Verification items for the finished model (mm, model axes). Coordinates: 2 decimals unless noted, no trailing zeros. Write each loop counter-clockwise with the first axis right and the second up, starting at its lowest first coordinate (ties: lowest second). Pieces come first, ordered by that corner, then holes. Notation, with made-up numbers: (-0.75, 52) -> (32.25, 52) arc R7 cw to (32.25, 61) -> close; hole circle Ø6 at (38, -9). An arc over 180 degrees is marked (long way). Write item = value, one per line. Start each with the question number.
(1) Gauge pin test, flat ends, axial feed: pin 1 Ø1.5 at (x, y) = (46.5, 2) entering from +Z; pin 2 Ø10 at (x, z) = (-20.5, 9) entering from -Y; pin 3 Ø0.8 at (x, y) = (93.5, 3) entering from +Z; pin 4 Ø2 at (x, y) = (74.5, 4) entering from -Z. Record the tip position at first contact, or that the pin passes through.
(2) Section check B-B (y = 6.5). State how many separate pieces and enclosed holes the cut face has, plus the area to 3 significant figures.
(3) Section check A-A (x = 58.5). Record the cut outline in (y, z), plus the area to 3 significant figures.
(4) Material ranges on probe 1 along X at (y, z) = (7.3, 0); probe 2 along X at (y, z) = (8, -33.5); probe 3 along Z at (x, y) = (-19, 4.5), recorded low to high. Write a range as [from, to].
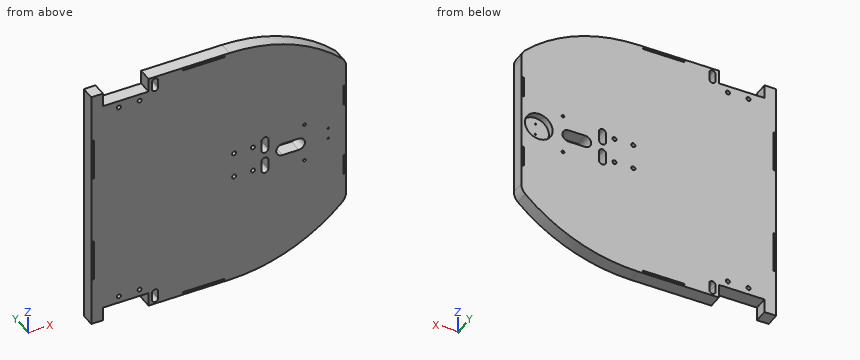
```python
from build123d import *

# Parameters (mm, degrees)
BOSS_EXTRUDE1_DEPTH = 10
SKETCH2_R           = 1
SKETCH2_R_2         = 1.5
SKETCH2_W           = 33
SKETCH2_H           = 10
CUT_EXTRUDE2_DEPTH  = 15
SKETCH3_R           = 10
CUT_EXTRUDE3_DEPTH  = 5
CUT_EXTRUDE4_DEPTH  = 15
SKETCH5_W           = 30
SKETCH5_H           = 1
SKETCH5_W_2         = 1
SKETCH5_H_2         = 30
SKETCH5_H_3         = 15
CUT_EXTRUDE6_DEPTH  = 15
SKETCH6_R           = 0.5
CUT_EXTRUDE7_DEPTH  = 15
SKETCH7_R           = 1.5
CUT_EXTRUDE8_DEPTH  = 132.376296717


with BuildPart() as part:
    # Sketch1 → Boss-Extrude1 (new body)
    with BuildSketch(Plane(origin=(0, 0, 0), x_dir=(1, 0, 0), z_dir=(0, 1, 0))):
        with BuildLine():
            Line((-89.389143795, -90), (-89.389143795, 90))
            Line((-89.389143795, 90), (10.610856205, 90))
            ThreePointArc((10.610856205, 90), (54.533138364, 81.496268076), (92.107774725, 57.214031174))
            ThreePointArc((92.107774725, 57.214031174), (94.381847518, 53.920998768), (95.182620993, 50))
            Line((95.182620993, 50), (95.182620993, -50))
            ThreePointArc((95.182620993, -50), (94.381847518, -53.920998768), (92.107774725, -57.214031174))
            ThreePointArc((92.107774725, -57.214031174), (54.533138364, -81.496268076), (10.610856205, -90))
            Line((10.610856205, -90), (-89.389143795, -90))
        make_face()
    extrude(amount=BOSS_EXTRUDE1_DEPTH)

    # Sketch2 → Cut-Extrude2 (cut, symmetric)
    with BuildSketch(Plane(origin=(0, 10, 0), x_dir=(1, 0, 0), z_dir=(0, 1, 0))):
        with Locations(Location((65, 14.131573434, 0), (0, 0, 90))):
            Circle(SKETCH2_R)
        with Locations(Location((27.688972694, 9.173126615, 0), (0, 0, 90))):
            Circle(SKETCH2_R_2)
        with Locations(Location((14.053243942, 9.173126615, 0), (0, 0, 90))):
            Circle(SKETCH2_R_2)
        with Locations(Location((14.053243942, -9.173126615, 0), (0, 0, 90))):
            Circle(SKETCH2_R_2)
        with Locations(Location((27.688972694, -9.173126615, 0), (0, 0, 90))):
            Circle(SKETCH2_R_2)
        with Locations(Location((65, -14.131573434, 0), (0, 0, 90))):
            Circle(SKETCH2_R)
        with BuildLine():
            Line((-40.968894473, 86.42714575), (-40.968894473, 80.97285425))
            ThreePointArc((-40.968894473, 80.97285425), (-43.204350858, 78.737397865), (-45.439807243, 80.97285425))
            Line((-45.439807243, 80.97285425), (-45.439807243, 86.42714575))
            ThreePointArc((-45.439807243, 86.42714575), (-43.204350858, 88.662602135), (-40.968894473, 86.42714575))
        make_face()
        with BuildLine():
            Line((38.845478036, 11.594873944), (38.845478036, 4.405126056))
            ThreePointArc((38.845478036, 4.405126056), (36.366254627, 1.925902647), (33.887031217, 4.405126056))
            Line((33.887031217, 4.405126056), (33.887031217, 11.594873944))
            ThreePointArc((33.887031217, 11.594873944), (36.366254627, 14.074097353), (38.845478036, 11.594873944))
        make_face()
        with Locations((-64.401012641, 85)):
            Rectangle(SKETCH2_W, SKETCH2_H)
        with BuildLine():
            Line((38.845478036, -11.594873944), (38.845478036, -4.405126056))
            ThreePointArc((38.845478036, -4.405126056), (36.366254627, -1.925902647), (33.887031217, -4.405126056))
            Line((33.887031217, -4.405126056), (33.887031217, -11.594873944))
            ThreePointArc((33.887031217, -11.594873944), (36.366254627, -14.074097353), (38.845478036, -11.594873944))
        make_face()
        with BuildLine():
            Line((-40.968894473, -86.42714575), (-40.968894473, -80.97285425))
            ThreePointArc((-40.968894473, -80.97285425), (-43.204350858, -78.737397865), (-45.439807243, -80.97285425))
            Line((-45.439807243, -80.97285425), (-45.439807243, -86.42714575))
            ThreePointArc((-45.439807243, -86.42714575), (-43.204350858, -88.662602135), (-40.968894473, -86.42714575))
        make_face()
        with Locations((-64.401012641, -85)):
            Rectangle(SKETCH2_W, SKETCH2_H)
    extrude(amount=CUT_EXTRUDE2_DEPTH, both=True, mode=Mode.SUBTRACT)

    # Sketch3 → Cut-Extrude3 (cut, symmetric)
    with BuildSketch(Plane(origin=(0, 10, 0), x_dir=(1, 0, 0), z_dir=(0, 1, 0))):
        with Locations(Location((82.479810043, 0, 0), (0, 0, 270))):
            Circle(SKETCH3_R)
    extrude(amount=CUT_EXTRUDE3_DEPTH, both=True, mode=Mode.SUBTRACT)

    # Sketch4 → Cut-Extrude4 (cut, symmetric)
    with BuildSketch(Plane(origin=(0, 10, 0), x_dir=(1, 0, 0), z_dir=(0, 1, 0))):
        with BuildLine():
            Line((49.010294015, 4.462602137), (60.91056638, 4.462602137))
            ThreePointArc((60.91056638, 4.462602137), (65.373168517, 0), (60.91056638, -4.462602137))
            Line((60.91056638, -4.462602137), (49.010294015, -4.462602137))
            ThreePointArc((49.010294015, -4.462602137), (44.547691878, 0), (49.010294015, 4.462602137))
        make_face()
    extrude(amount=CUT_EXTRUDE4_DEPTH, both=True, mode=Mode.SUBTRACT)

    # Sketch5 → Cut-Extrude6 (cut, symmetric)
    with BuildSketch(Plane(origin=(0, 10, 0), x_dir=(1, 0, 0), z_dir=(0, 1, 0))):
        with Locations((-7.901012641, 88.5)):
            Rectangle(SKETCH5_W, SKETCH5_H)
        with Locations((-87.889143795, 40)):
            Rectangle(SKETCH5_W_2, SKETCH5_H_2)
        with Locations((93.682620993, 27.5)):
            Rectangle(SKETCH5_W_2, SKETCH5_H_3)
        with Locations((93.682620993, -27.5)):
            Rectangle(SKETCH5_W_2, SKETCH5_H_3)
        with Locations((-7.901012641, -88.5)):
            Rectangle(SKETCH5_W, SKETCH5_H)
        with Locations((-87.889143795, -40)):
            Rectangle(SKETCH5_W_2, SKETCH5_H_2)
    extrude(amount=CUT_EXTRUDE6_DEPTH, both=True, mode=Mode.SUBTRACT)

    # Sketch6 → Cut-Extrude7 (cut, symmetric)
    with BuildSketch(Plane(origin=(0, 5, 0), x_dir=(1, 0, 0), z_dir=(0, 1, 0))):
        with Locations(Location((82.244112685, 2.835581496, 0), (0, 0, 270))):
            Circle(SKETCH6_R)
        with Locations(Location((82.244112685, -5.164418504, 0), (0, 0, 270))):
            Circle(SKETCH6_R)
    extrude(amount=CUT_EXTRUDE7_DEPTH, both=True, mode=Mode.SUBTRACT)

    # Sketch7 → Cut-Extrude8 (cut, through all)
    with BuildSketch(Plane(origin=(0, 10, 0), x_dir=(1, 0, 0), z_dir=(0, 1, 0))):
        with Locations(Location((-69.389143795, 75, 0), (0, 0, 270))):
            Circle(SKETCH7_R)
        with Locations(Location((-54.389143795, 75, 0), (0, 0, 270))):
            Circle(SKETCH7_R)
        with Locations(Location((-69.389143795, -75, 0), (0, 0, 270))):
            Circle(SKETCH7_R)
        with Locations(Location((-54.389143795, -75, 0), (0, 0, 270))):
            Circle(SKETCH7_R)
    extrude(amount=-CUT_EXTRUDE8_DEPTH, mode=Mode.SUBTRACT)


solid = part.part
```
Response:
q1.pin_1 = 84.63
q1.pin_2 = 0
q1.pin_3 = 56.11
q1.pin_4 = -71.79
q2.separate_pieces = 1
q2.enclosed_holes = 22
q2.area = 29,800 mm2
q3.outline = (0, -79.82) -> (10, -79.82) -> (10, -4.46) -> (0, -4.46) -> close; (0, 4.46) -> (10, 4.46) -> (10, 79.82) -> (0, 79.82) -> close
q3.area = 1,510 mm2
q4.probe_1 = [-89.39, 44.55], [65.37, 72.48], [92.48, 95.18]
q4.probe_2 = [-89.39, -88.39], [-87.39, 93.18], [94.18, 95.18]
q4.probe_3 = [-90, -89], [-88, 88], [89, 90]
